Verification items for the finished model (mm, model axes). A direction names the side the tool comes from. Coordinates: 2 decimals unless noted, no trailing zeros. Loops run counter-clockwise (first coordinate to the right, second up) from the corner with the lowest first, then second, coordinate; pieces in that order, holes last. Notation, with made-up numbers: (58.5, -6) - (80.5, -6) arc R18 cw to (80.5, 9) - close; hole circle Ø5 at (-24, 40.25). An arc over 180 degrees is marked (long way). One line per item, written item: value. Start each with the question number.
(1) Section check D-D (z = -84.5). Record the boundary of the cut face in (x, y) (3 decimals), plus the area to 3 significant figures.
(2) Draft check along X on faces 4 (the face through (99, -3.175, -96)), 5 (the face through (52, 13, -195)), 6 (the face through (39, -2, -178)), 7 (the face through (-3.175, 11, -99)). Enter one of: +X half, -X half, draft (parallel to the pull), parting line (faces both ways), or undercut.
(3) Section check C-C (x = 40.5). Record the boundary of the cut face in (y, z) (3 decimals).
(4) Section check A-A (y = 8.5). Record the boundary of the cut face in (x, z) (3 decimals), plus the area to 3 significant figures.
(5) Section check B-B (z = -166.5). Record the boundary of the cut face in (x, y) (3 decimals).
(6) Set-up check for faces 1 (the face through (96, 13, 0)), 2 (the face through (32.014, 9, -196)), 3 (the face through (41.167, -1.61, -38.461)): record each of +Z, -Z, +X, -X, +Y, -Y from which the full face is reachable in a straight line by a thin tool's end or side.
(7) Thickness scan on probe 1 along X at (y, z) = (-1.7, -185) (3 decimals); probe 2 along X at (y, z) = (7, -79) (3 decimals); probe 3 along Z at (x, y) = (20, 21.5) (3 decimals). Record the ranges inside material, lowest first. Write a range as [from, to].
(8) Gauge pin test, flat ends, axial feed: P1, Ø15, axis at x = 19.51, z = -185, coming from the +Y side; P2, Ø1, axis at x = 107.5, y = -1.5, coming from the -Z side. Record the tip position at first contact, or that the pin passes through.
Autodesk Inventor part; units mm, degrees
ref_plane "YZ Plane" through (0, 0, 0) normal (1, 0, 0) x (0, 1, 0)
ref_plane "XZ Plane" through (0, 0, 0) normal (0, 1, 0) x (-1, 0, 0)
ref_plane "XY Plane" through (0, 0, 0) normal (0, 0, 1) x (1, 0, 0)
sketch "Sketch1" plane through (0, 0, 0) normal (0, 1, 0) x (-1, 0, 0)
  line L0 (0, 0) -> (-195, 0)
  line L1 (-195, 0) -> (-195, -195)
  line L2 (-195, -195) -> (0, -195)
  line L3 (0, -195) -> (0, 0)
  line L4 (3.175, 3.175) -> (-198.1708, 3.175)
  line L5 (-198.1708, 3.175) -> (-198.1708, -198.1708)
  line L6 (-198.1708, -198.1708) -> (3.175, -198.1708)
  line L7 (3.175, -198.1708) -> (3.175, 3.175)
  dimension "d0" = 195
  dimension "d1" = 195
  dimension "d2" = 201.3458
  dimension "d3" = 201.3458
extrude "Extrusion1" add sketch "Sketch1" along normal blind 25.4
sketch "Sketch2" plane through (0, 0, 0) normal (0, 1, 0) x (-1, 0, 0)
  line L0 (3.175, 3.175) -> (-198.1708, 3.175)
  line L1 (3.175, -198.1708) -> (3.175, 3.175)
  line L2 (-198.1708, 3.175) -> (-198.1708, -198.1708)
  line L3 (-198.1708, -198.1708) -> (3.175, -198.1708)
  point P0 (0, 0)
extrude "Extrusion2" add sketch "Sketch2" against normal blind 3.175
sketch "Sketch3" plane through (0, 0, 0) normal (0, 1, 0) x (1, 0, 0)
  line L0 (0, 195) -> (195, 195)
  line L1 (0, 195) -> (97.4979, 195)
  line L2 (97.4979, 195) -> (136.4979, 195)
  line L3 (97.4979, 195) -> (136.4979, 195) construction
  line L4 (136.4979, 195) -> (58.5199, 195)
  line L5 (58.5199, 195) -> (58.5199, 117.022)
  line L6 (58.5199, 117.022) -> (136.4979, 117.022)
  line L7 (136.4979, 117.022) -> (136.4979, 195)
  point P0 (0, 0)
  dimension "d8" = 97.4979
  dimension "d9" = 39
  dimension "d10" = 0
  dimension "d11" = 77.978
  dimension "d12" = 77.978
extrude "Extrusion3" cut sketch "Sketch3" against normal blind 3.175
sketch "Sketch4" plane through (0, 0, 0) normal (0, 1, 0) x (1, 0, 0)
  line L0 (0, 0) -> (0, 195)
  line L1 (0, 195) -> (195, 195)
  line L2 (58.5199, 117.022) -> (58.5199, 195)
  line L3 (136.4979, 195) -> (136.4979, 117.022)
  line L4 (195, 195) -> (195, 0)
  line L5 (0, 0) -> (0, 195)
  line L6 (0, 195) -> (19.5072, 195)
  line L7 (19.5072, 195) -> (39.0144, 195)
  line L8 (0, 195) -> (0, 185)
  circle A0 centre (19.5072, 185) radius 6.5
  circle A1 centre (39.0144, 185) radius 7
  line L9 (136.4979, 195) -> (195, 195)
  line L10 (195, 195) -> (195, 184.9924)
  line L11 (198.1708, 198.1708) -> (198.1708, -3.175)
  line L12 (195, 195) -> (205.0076, 195) construction
  line L13 (195, 195) -> (175.4928, 195)
  line L14 (195, 195) -> (214.5072, 195) construction
  line L15 (175.4928, 195) -> (155.9856, 195)
  circle A2 centre (175.4928, 184.9924) radius 6.5024
  circle A3 centre (155.9856, 184.9924) radius 6.9977
  dimension "d15" = 58.5199
  dimension "d16" = 19.5072
  dimension "d17" = 19.5072
  dimension "d18" = 10
  dimension "d19" = 13
  dimension "d20" = 14
  dimension "d21" = 10.0076
  dimension "d22" = 90
  dimension "d23" = 19.5072
  dimension "d24" = 180
  dimension "d25" = 19.5072
  dimension "d26" = 13.0048
  dimension "d27" = 13.9954
extrude "Extrusion4" cut sketch "Sketch4" against normal blind 3.175
sketch "Sketch5" plane through (0, -3.175, 0) normal (0, -1, 0) x (1, 0, 0)
  circle A0 centre (61.0901, -58.3837) radius 57.15
  line L0 (61.0901, -58.3837) -> (61.0901, -1.2337)
  line L1 (61.0901, -58.3837) -> (118.2401, -58.3837) construction
  line L2 (61.0901, -58.3837) -> (20.679, -17.9725)
  line L3 (61.0901, -58.3837) -> (118.2401, -58.3837) construction
  point P0 (0, 0)
  dimension "d32" = 114.3
  dimension "d33" = 57.15
  dimension "d34" = 90
  dimension "d35" = 57.15
  dimension "d36" = 135
extrude "Extrusion5" cut sketch "Sketch5" against normal blind 3.175 contours L0 L2 A0 picked at (52.2233, -21.4506)
sketch "Sketch6" plane through (0, -3.175, 0) normal (0, -1, 0) x (1, 0, 0)
  line L0 (136.4979, -195) -> (58.5199, -195)
  line L1 (-3.175, -198.1708) -> (198.1708, -198.1708)
  line L2 (136.4979, -195) -> (58.5199, -195)
  line L3 (58.5199, -195) -> (58.5199, -198.175)
  line L4 (58.5199, -198.175) -> (136.4979, -198.175)
  line L5 (136.4979, -198.175) -> (136.4979, -195)
  point P0 (0, 0)
  point P1 (136.4979, -198.1708)
  point P2 (58.5199, -198.1708)
  dimension "d39" = 3.175
extrude "Extrusion6" cut sketch "Sketch6" against normal through all contours L5 L1 L3 L0
sketch "Sketch7" plane through (0, -3.175, 0) normal (0, -1, 0) x (1, 0, 0)
  circle A0 centre (39.0144, -185) radius 7
  line L0 (58.5199, -198.1708) -> (-3.175, -198.1708)
  line L1 (32.0144, -185) -> (46.0098, -185)
  line L2 (46.0098, -185) -> (46.0098, -198.1708)
  line L3 (46.0098, -198.1708) -> (32.0144, -198.1708)
  line L4 (32.0144, -198.1708) -> (32.0144, -185)
  point P0 (0, 0)
  dimension "d42" = 13.9954
extrude "Extrusion7" cut sketch "Sketch7" against normal through all contours L1 L2 A0 | A0 L2 L0 L4 picked at (36.7458, -185.5521)
properties part number "FixedLid"
Responses:
1. outline: (-3.175, -3.175) - (198.171, -3.175) - (198.171, 25.4) - (195, 25.4) - (195, 0) - (0, 0) - (0, 25.4) - (-3.175, 25.4) - close
1. area: 800 mm²
2. face 4: draft
2. face 5: undercut
2. face 6: undercut
2. face 7: -X half
3. outline: (-3.175, -178.159) - (0, -178.159) - (0, -37.794) - (-3.175, -37.794) - close; (-3.175, -5.072) - (0, -5.072) - (0, 0) - (25.4, 0) - (25.4, 3.175) - (-3.175, 3.175) - close
4. outline: (-3.175, -198.171) - (32.014, -198.171) - (32.014, -195) - (0, -195) - (0, 0) - (195, 0) - (195, -195) - (136.498, -195) - (136.498, -198.171) - (198.171, -198.171) - (198.171, 3.175) - (-3.175, 3.175) - close; (46.01, -198.171) - (58.52, -198.171) - (58.52, -195) - (46.01, -195) - close
4. area: 2,220 mm²
5. outline: (-3.175, -3.175) - (58.52, -3.175) - (58.52, 0) - (0, 0) - (0, 25.4) - (-3.175, 25.4) - close; (136.498, -3.175) - (198.171, -3.175) - (198.171, 25.4) - (195, 25.4) - (195, 0) - (136.498, 0) - close
6. face 1: +Y
6. face 2: -Z, +Y, -Y
6. face 3: +Y, -Y
7. probe 1: x = [-3.175, 13.007], [26.007, 32.014], [46.014, 58.52], [136.498, 148.988], [162.983, 168.99], [181.995, 198.171]
7. probe 2: x = [-3.175, 0], [195, 198.171]
7. probe 3: z = [-198.171, -195], [0, 3.175]
8. P1: stops at y = 0
8. P2: stops at z = -117.02
